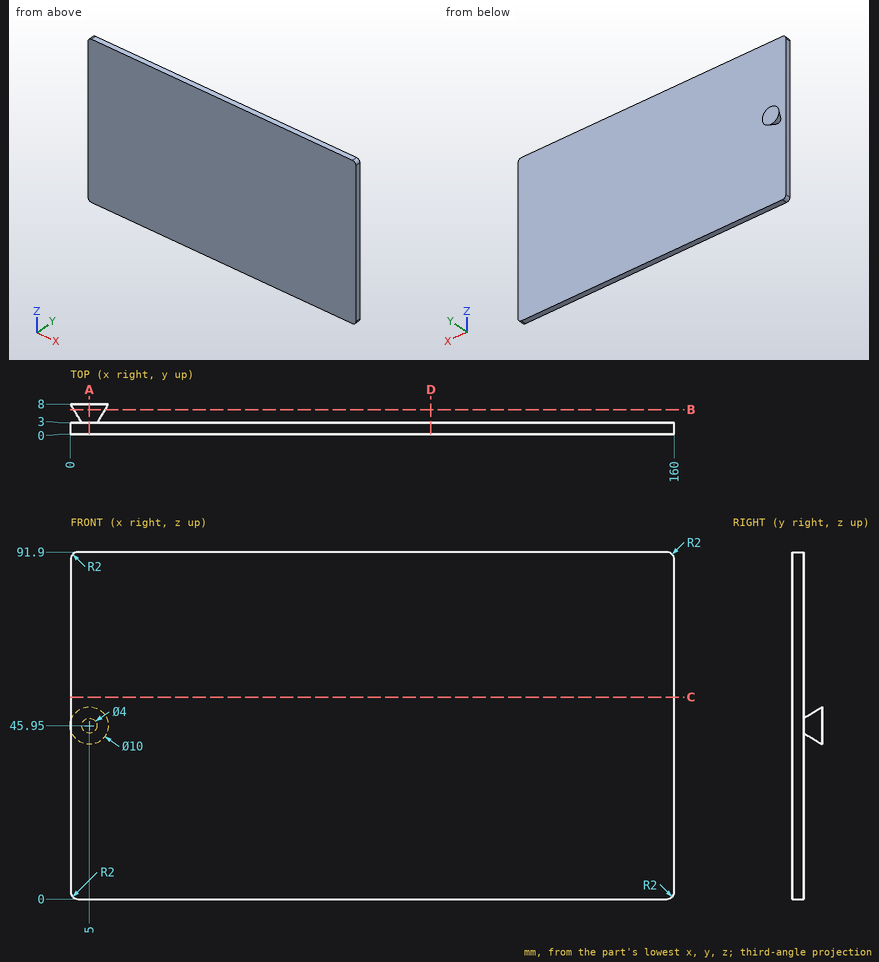
Source: three-view drawing plus pictorial views. Frame: mm from the lowest corner of the part. Give positions to 0.01 mm unless a question says otherwise; leave off trailing zeros. Order: outer loops, then holes, each group sorted by start corner. A loop starts at its lowest first (then second) coordinate and runs counter-clockwise, first axis right, second up. Notation, with made-up numbers: (85, 89.5) -> (123, 89.5) arc R18 cw to (123, 94.5) -> close; hole circle Ø8 at (85.25, 32). An arc over 180 degrees is marked (long way). Put each result on its own line as item: value.
Q1. Section A-A, the plane x = 5. Return loops of the section in (y, z), then the cut area to 3 significant figures.
Here are the results:
outline: (0, 0) -> (3, 0) -> (3, 43.95) -> (8, 40.95) -> (8, 50.95) -> (3, 47.95) -> (3, 91.9) -> (0, 91.9) -> close
area: 311 mm^2
Q2. Section C-C, the plane z = 53.5. Return loops of the section in (x, y).
Here are the results:
outline: (0, 0) -> (160, 0) -> (160, 3) -> (0, 3) -> close
Q3. Section D-D, the plane x = 95.5. Return loops of the section in (y, z), then the cut area to 3 significant figures.
Here are the results:
outline: (0, 0) -> (3, 0) -> (3, 91.9) -> (0, 91.9) -> close
area: 276 mm^2
Q4. Pin query (flat end, axial travel): pin 1 (1.5 mm diameter, centred on x = 29, z = 61, fed in from +Y). Return the tip coordinate at first contact, or that it passes through.
Here are the results:
pin 1: stops at y = 3
Q5. Section B-B, the plane y = 6.5. Return loops of the section in (x, z).
Here are the results:
outline: circle Ø8.2 at (5, 45.95)
Q6. Material intervals for L1, parallel to Y at x = 50, z = 69; L2, parallel to X at y = 5, z = 45; L3, parallel to X at y = 6, z = 47.5, sorted ascending.
Here are the results:
L1: y = 0 to 3
L2: x = 1.94 to 8.06
L3: x = 1.53 to 8.47
